Can you work these out from the model? Positions are in its coordinate system, mm. A direction names the side the tool comes from. Give positions to 0.01 mm unless a question says otherwise; leave off trailing zeros. Loops run counter-clockwise (first coordinate to the right, second up) from the corner with the lowest first, then second, coordinate; pieces in that order, holes last. Notation, with made-up numbers: (-23, 22.25) - (-14, 22.25) arc R34 ccw to (-14, 60.25) - close; hole circle Ø9 at (5, 58). An arc over 180 degrees is marked (long way). Use a Markdown table: item, result. Add a question column.
Autodesk Inventor part; units mm, degrees
ref_plane "YZ Plane" through (0, 0, 0) normal (1, 0, 0) x (0, 1, 0)
ref_plane "XZ Plane" through (0, 0, 0) normal (0, 1, 0) x (-1, 0, 0)
ref_plane "XY Plane" through (0, 0, 0) normal (0, 0, 1) x (1, 0, 0)
sketch "Sketch1" plane through (0, 0, 0) normal (0, 1, 0) x (-1, 0, 0)
  line L0 (0, 0) -> (145, 0)
  line L1 (145, 0) -> (145, -15)
  line L2 (145, -15) -> (0, -15)
  line L3 (0, -15) -> (0, 0)
  dimension "d0" = 145
  dimension "d1" = 15
extrude "Extrusion1" add sketch "Sketch1" along normal blind 3
sketch "Sketch2" plane through (0, 3, 0) normal (0, 1, 0) x (1, 0, 0)
  line L0 (-145, 0) -> (0, 0)
  line L1 (0, 15) -> (-145, 15)
  line L2 (-145, 0) -> (-139, 0)
  line L3 (-139, 0) -> (-139, 15)
  line L4 (-139, 15) -> (-145, 15)
  line L5 (-145, 15) -> (-145, 0)
  line L6 (0, 0) -> (-6, 0)
  line L7 (-6, 0) -> (-6, 15)
  line L8 (-6, 15) -> (0, 15)
  line L9 (0, 15) -> (0, 0)
  dimension "d4" = 6
  dimension "d5" = 6
extrude "Extrusion2" add sketch "Sketch2" along normal blind 20 contours L5 L1 L3 L0 | L7 L1 L9 L0
sketch "Sketch3" plane through (0, 0, 0) normal (1, 0, 0) x (0, 0, -1)
  line L0 (0, 3) -> (15, 3) construction
  line L1 (7.5, 3) -> (7.5, 15.5) construction
  circle A0 centre (7.5, 15.5) radius 5
  point P0 (0, 0)
  dimension "d8" = 12.5
  dimension "d9" = 10
extrude "Extrusion3" cut sketch "Sketch3" against normal blind 156
sketch "Sketch4" plane through (-139, 3, 0) normal (1, 0, 0) x (0, 0, -1)
  circle A0 centre (7.5, 12.5) radius 5
  circle A1 centre (7.5, 12.5) radius 5
  circle A2 centre (7.5, 12.5) radius 5
  circle A3 centre (7.5, 12.5) radius 2.5
  point P0 (0, -3)
  dimension "d12" = 5
extrude "Extrusion4" add sketch "Sketch4" against normal blind 1.5
sketch "Sketch5" plane through (-6, 3, -15) normal (-1, 0, 0) x (0, 0, 1)
  circle A0 centre (7.5, 12.5) radius 2.5
  circle A1 centre (7.5, 12.5) radius 5
  circle A2 centre (7.5, 12.5) radius 2.4999
  point P0 (15, -3)
extrude "Extrusion5" add sketch "Sketch5" against normal blind 1.5
sketch "Sketch6" plane through (0, 3, 0) normal (0, 1, 0) x (1, 0, 0)
  line L0 (0, 0) -> (-145, 0)
  line L1 (-72.5, 0) -> (-76.5, 0)
  line L2 (-76.5, 0) -> (-76.5, -4)
  line L3 (-76.5, -4) -> (-72.5, -4)
  line L4 (-72.5, -4) -> (-72.5, 0)
  line L5 (-72.5, 0) -> (-68.5, 0)
  line L6 (-68.5, 0) -> (-68.5, -4)
  line L7 (-68.5, -4) -> (-72.5, -4)
  line L8 (-72.5, -4) -> (-72.5, 0)
  dimension "d17" = 4
  dimension "d18" = 4
  dimension "d19" = 4
extrude "Extrusion6" add sketch "Sketch6" against normal blind 3
sketch "Sketch7" plane through (0, 3, 0) normal (0, 1, 0) x (1, 0, 0)
  circle A0 centre (-72.5, 0) radius 3.2
  line L0 (-68.5, 0) -> (-68.5, -4)
  line L1 (-68.5, -4) -> (-76.5, -4)
  line L2 (-76.5, -4) -> (-76.5, 4)
  line L3 (-76.5, 4) -> (-68.5, 4)
  line L4 (-68.5, 4) -> (-68.5, -4)
  point P0 (0, 0)
  dimension "d22" = 6.4
  dimension "d23" = 8
extrude "Extrusion7" add sketch "Sketch7" against normal blind 10
sketch "Sketch8" plane through (-72.5, 0, 0) normal (0, -1, 0) x (1, 0, 0)
  point P0 (72.5, 0)
sketch "Sketch9" plane through (-72.5, 0, 0) normal (0, -1, 0) x (1, 0, 0)
  circle A0 centre (0, 0) radius 3.2
  point P0 (72.5, 0)
extrude "Extrusion8" cut sketch "Sketch9" against normal blind 7.5
sketch "Sketch10" plane through (0, 0, 0) normal (0, -1, 0) x (1, 0, 0)
  line L0 (0, 0) -> (0, -15) construction
  line L1 (0, 0) -> (-16, 0) construction
  line L2 (-16, 0) -> (-16, -25) construction
  line L3 (-16, -25) -> (0, -25) construction
  line L4 (0, -25) -> (0, 0) construction
  line L5 (-145, -15) -> (-145, 0) construction
  line L6 (-145, 0) -> (-129, 0) construction
  line L7 (-129, 0) -> (-129, -25) construction
  line L8 (-129, -25) -> (-145, -25) construction
  line L9 (-145, -25) -> (-145, 0) construction
  line L10 (0, -25) -> (-2, -25)
  line L11 (-2, -25) -> (-2, -2)
  line L12 (-2, -2) -> (-14, -2)
  line L13 (-14, -2) -> (-14, -25)
  line L14 (-16, -25) -> (-16, 0)
  line L15 (-68.5, 0) -> (-6, 0)
  line L16 (-6, 0) -> (0, 0)
  line L17 (0, 0) -> (-16, 0)
  line L18 (0, -25) -> (0, 0)
  line L19 (0, -2.5) -> (-4.5, -2.5)
  line L20 (-129, -25) -> (-129, 0)
  line L21 (-145, 0) -> (-139, 0)
  line L22 (-145, 0) -> (-145, -25)
  line L23 (-145, -25) -> (-143, -25)
  line L24 (-143, -25) -> (-143, -2)
  line L25 (-143, -2) -> (-131, -2)
  line L26 (-131, -2) -> (-131, -25)
  line L27 (-129, -25) -> (-131, -25)
  line L28 (-14, -25) -> (-16, -25)
  line L29 (-129, 0) -> (-145, 0)
  dimension "d28" = 16
  dimension "d29" = 25
  dimension "d30" = 16
  dimension "d31" = 25
  dimension "d32" = 2
  dimension "d33" = 23
  dimension "d34" = 12
  dimension "d35" = 2
  dimension "d36" = 23
  dimension "d37" = 12
extrude "Extrusion9" add sketch "Sketch10" along normal blind 3.5
sketch "Sketch11" plane through (0, 0, 0) normal (0, 1, 0) x (1, 0, 0)
  line L0 (0, 25) -> (0, 0)
  line L1 (-16, 0) -> (-16, 25)
  line L2 (0, 25) -> (-16, 25)
  line L3 (-16, 25) -> (-16, 15.0002)
  line L4 (-16, 15.0002) -> (0, 15.0002)
  line L5 (0, 15.0002) -> (0, 25)
  line L6 (-131, 25) -> (-129, 25)
  line L7 (-145, 0) -> (-145, 25)
  line L8 (-129, 25) -> (-145, 25)
  line L9 (-145, 25) -> (-145, 15.0002)
  line L10 (-145, 15.0002) -> (-129, 15.0002)
  line L11 (-129, 15.0002) -> (-129, 25)
extrude "Extrusion10" add sketch "Sketch11" along normal blind 3
sketch "Sketch12" plane through (0, -3.5, 0) normal (0, -1, 0) x (1, 0, 0)
  line L0 (0, -25) -> (0, 0)
  line L1 (0, 0) -> (-16, 0)
  line L2 (0, -25) -> (-4, -25)
  line L3 (-4, -25) -> (-4, 0)
  line L4 (-4, 0) -> (0, 0)
  line L5 (0, 0) -> (0, -25)
  line L6 (-16, 0) -> (-16, -25)
  line L7 (0, 0) -> (-16, 0)
  line L8 (-16, 0) -> (-16, -4)
  line L9 (-16, -4) -> (0, -4)
  line L10 (0, -4) -> (0, 0)
  line L11 (-16, -25) -> (-12, -25)
  line L12 (-12, -25) -> (-12, 0)
  line L13 (-12, 0) -> (-16, 0)
  line L14 (-16, 0) -> (-16, -25)
  line L15 (-129, 0) -> (-145, 0)
  line L16 (-129, -25) -> (-133, -25)
  line L17 (-133, -25) -> (-133, 0)
  line L18 (-133, 0) -> (-129, 0)
  line L19 (-129, 0) -> (-129, -25)
  line L20 (-145, -25) -> (-143, -25)
  line L21 (-145, -25) -> (-141, -25)
  line L22 (-141, -25) -> (-141, 0)
  line L23 (-141, 0) -> (-145, 0)
  line L24 (-145, 0) -> (-145, -25)
  line L25 (-129, 0) -> (-145, 0)
  line L26 (-145, 0) -> (-145, -4)
  line L27 (-145, -4) -> (-129, -4)
  line L28 (-129, -4) -> (-129, 0)
  dimension "d42" = 4
  dimension "d43" = 4
  dimension "d44" = 4
  dimension "d45" = 4
  dimension "d46" = 4
extrude "Extrusion11" add sketch "Sketch12" along normal blind 2
sketch "Sketch13" plane through (-2, 0, -25) normal (0, 0, -1) x (-1, 0, 0)
  line L0 (-2, 3) -> (14, 3)
  line L1 (2, -5.5) -> (-2, -5.5)
  line L2 (-2, 3) -> (0, 3)
  line L3 (0, 3) -> (0, -5.5)
  line L4 (0, -5.5) -> (-2, -5.5)
  line L5 (-2, -5.5) -> (-2, 3)
  line L6 (0, 0) -> (0, -3.5)
  line L7 (2, -5.5) -> (0, -5.5)
  line L8 (0, -5.5) -> (0, -3.5)
  line L9 (0, -3.5) -> (2, -3.5)
  line L10 (2, -3.5) -> (2, -5.5)
  line L11 (14, -5.5) -> (10, -5.5)
  line L12 (10, -3.5) -> (14, -3.5)
  line L13 (14, -3.5) -> (14, -5.5)
  line L14 (14, -5.5) -> (10, -5.5)
  line L15 (10, -5.5) -> (10, -3.5)
  line L16 (66.5, 3) -> (4, 3)
  line L17 (14, -3.5) -> (12, -3.5)
  line L18 (12, -3.5) -> (12, 3)
  line L19 (12, 3) -> (14, 3)
  line L20 (14, 3) -> (14, -3.5)
  line L21 (0, 0) -> (12, 0)
  line L22 (12, 3) -> (0, 3)
  line L23 (0, 3) -> (0, 0)
  line L24 (0, 0) -> (12, 0)
  line L25 (12, 0) -> (12, 3)
  line L26 (127, 0) -> (127, 3)
  line L27 (143, 3) -> (143, -5.5)
  line L28 (127, 3) -> (143, 3)
  line L29 (143, 3) -> (143, 0)
  line L30 (143, 0) -> (127, 0)
  line L31 (127, 0) -> (127, 3)
  line L32 (143, -5.5) -> (139, -5.5)
  line L33 (143, 0) -> (141, 0)
  line L34 (141, 0) -> (141, -5.5)
  line L35 (141, -5.5) -> (143, -5.5)
  line L36 (143, -5.5) -> (143, 0)
  line L37 (141, -3.5) -> (139, -3.5)
  line L38 (139, -3.5) -> (141, -3.5)
  line L39 (141, -3.5) -> (141, -5.5)
  line L40 (141, -5.5) -> (139, -5.5)
  line L41 (139, -5.5) -> (139, -3.5)
  line L42 (127, 0) -> (14, 0)
  line L43 (131, -5.5) -> (127, -5.5)
  line L44 (127, 0) -> (129, 0)
  line L45 (129, 0) -> (129, -5.5)
  line L46 (129, -5.5) -> (127, -5.5)
  line L47 (127, -5.5) -> (127, 0)
  line L48 (131, -3.5) -> (131, -5.5)
  line L49 (131, -3.5) -> (129, -3.5)
  line L50 (129, -3.5) -> (129, -5.5)
  line L51 (129, -5.5) -> (131, -5.5)
  line L52 (131, -5.5) -> (131, -3.5)
  point P0 (-2, 0)
extrude "Extrusion12" add sketch "Sketch13" along normal blind 15 and the other way blind 16.5
sketch "Sketch14" plane through (-145, 3, -15) normal (-1, 0, 0) x (0, 0, 1)
  circle A0 centre (7.5, 12.5) radius 2.5
  circle A1 centre (7.5, 12.5) radius 5.5
  point P0 (15, -3)
  dimension "d53" = 11
extrude "Extrusion13" cut sketch "Sketch14" against normal blind 4.5
sketch "Sketch15" plane through (0, 3, -15) normal (1, 0, 0) x (0, 0, -1)
  circle A0 centre (-7.5, 12.5) radius 5.5
  circle A1 centre (-7.5, 12.5) radius 5.5
  point P0 (-15, -3)
extrude "Extrusion14" cut sketch "Sketch15" against normal blind 4.5
properties part number "frontAxelHolder 9-1"
1. If we mould it in two halves opening along Y, with no side actions, what happens to faces 1 (the face through (-142.8, 10.6, -5)), 2 (the face through (-3, 23, -8)), 3 (the face through (-142, -5.5, -20))? For each: released by +Y, released by -Y, zero draft, split by the parting line, or undercut.
2. Suppose I cut it at D-D (z = -7.5). State how many separate pieces and enclosed holes the cut face has, and give its area (3 significant figures).
3. Suppose I cut it at A-A (z = -29). List the corners of the cut face in (x, y) for me.
4. Please list where these lines run through material, in increasing order: line 1 along X through (y, z) = (-2.5, -31); line 2 along Y through (x, z) = (-2.9, -7.5); line 3 along X through (y, z) = (1.25, -27). Write a range as [from, to].
5. Suppose I cut it at B-B (x = -72.5). List the corners of the cut face in (y, z) for me.
6. Suppose I cut it at C-C (y = 15.5). List the corners of the cut face in (x, z) for me.
7. On a 3-axis mill with a long thin cutter (end or side, diameter ignored), from which of +Z, -Z, +X, -X, +Y, -Y can I reach the whole of each face in a straight line? I mean faces 4 (the face through (-3, -5.5, -20)), 5 (the face through (-137, -2, -2)), 6 (the face through (-6, 13, -9)). Say none if no direction works.
8. Will these pins go through, and if not, where does the flat tip stop? P1, Ø9.5, axis at x = -7.5, z = -27, coming from the +Y side; P2, Ø5, axis at x = -136, z = -21.5, coming from the -Y side; P3, Ø2, axis at x = -71.5, y = -5, coming from the -Z side; P4, Ø0.6, axis at y = -5, z = -19, coming from the +X side.
Results below:
| question | item | result |
|---|---|---|
| 1 | face 1 | undercut |
| 1 | face 2 | released by +Y |
| 1 | face 3 | released by -Y |
| 2 | separate pieces | 3 |
| 2 | enclosed holes | 0 |
| 2 | area | 621 mm² |
| 3 | outline | (-145, -5.5) - (-141, -5.5) - (-141, -3.5) - (-143, -3.5) - (-143, 0) - (-131, 0) - (-131, -3.5) - (-133, -3.5) - (-133, -5.5) - (-129, -5.5) - (-129, 3) - (-145, 3) - close; (-16, -5.5) - (-12, -5.5) - (-12, -3.5) - (-14, -3.5) - (-14, 0) - (-2, 0) - (-2, -3.5) - (-4, -3.5) - (-4, -5.5) - (0, -5.5) - (0, 3) - (-16, 3) - close |
| 4 | line 1 | [-145, -143], [-131, -129], [-16, -14], [-2, 0] |
| 4 | line 2 | [-5.5, -3.5], [0, 10], [21, 23] |
| 4 | line 3 | [-145, -129], [-16, 0] |
| 5 | outline | (-7, -4) - (0, -4) - (0, -15) - (3, -15) - (3, -3.2) - (-7, -3.2) - close; (-7, 3.2) - (3, 3.2) - (3, 4) - (-7, 4) - close |
| 6 | outline | (-145, -15) - (-139, -15) - (-139, -10) - (-140.5, -10) - (-140.5, -13) - (-145, -13) - close; (-145, -2) - (-140.5, -2) - (-140.5, -5) - (-139, -5) - (-139, 0) - (-145, 0) - close; (-6, -15) - (0, -15) - (0, -13) - (-4.5, -13) - (-4.5, -10) - (-6, -10) - close; (-6, -5) - (-4.5, -5) - (-4.5, -2) - (0, -2) - (0, 0) - (-6, 0) - close |
| 7 | face 4 | +Z, -Z, +X, -Y |
| 7 | face 5 | -Z |
| 7 | face 6 | +Z, -Z, +Y |
| 8 | P1 | y = 3 |
| 8 | P2 | y = 0 |
| 8 | P3 | z = -4 |
| 8 | P4 | x = 0 |
